Read the model definition and answer for the solid it produces. Units are mm, in the model's axes. A direction names the side the tool comes from. Give positions to 0.01 mm unless a question says otherwise; leave off trailing zeros. Write each loop counter-clockwise with the first axis right and the second up, starting at its lowest first coordinate (ties: lowest second). Pieces come first, ordered by that corner, then holes.
```python
from build123d import *

# Parameters (mm, degrees)
BOSS_EXTRUDE1_DEPTH = 7
SKETCH3_R           = 4.2
SKETCH3_R_2         = 31
CUT_EXTRUDE1_DEPTH  = 156.951680739
SKETCH5_R           = 31
SKETCH5_R_2         = 29.4
BOSS_EXTRUDE3_DEPTH = 2
CUT_EXTRUDE3_DEPTH  = 156.951680739


with BuildPart() as part:
    # Sketch1 → Boss-Extrude1 (new, symmetric)
    with BuildSketch(Plane.XY):
        with BuildLine():
            Line((-41.457265734, 7.66555398), (-63.259986532, -110.249105832))
            ThreePointArc((-63.259986532, -110.249105832), (-57.764447863, -119.708474266), (-47.579981062, -115.713823794))
            Line((-47.579981062, -115.713823794), (-25.616732048, -74.324411645))
            ThreePointArc((-25.616732048, -74.324411645), (-5.909772036, -59.526451333), (18.065040544, -65.231910476))
            Line((18.065040544, -65.231910476), (84.767367566, -118.347513787))
            ThreePointArc((84.767367566, -118.347513787), (95.212080879, -118.36382677), (97.598433891, -108.195364664))
            Line((97.598433891, -108.195364664), (38.136901528, 17.973378699))
            ThreePointArc((38.136901528, 17.973378699), (-5.414703798, 41.810842885), (-41.457265734, 7.66555398))
        make_face()
    extrude(amount=BOSS_EXTRUDE1_DEPTH, both=True)

    # Sketch3 → Cut-Extrude1 (cut, through all)
    with BuildSketch(Plane.XY.offset(7)):
        with Locations((-55, -111.776398371)):
            Circle(SKETCH3_R)
        with Locations((90, -111.776398371)):
            Circle(SKETCH3_R)
        Circle(SKETCH3_R_2)
    extrude(amount=-CUT_EXTRUDE1_DEPTH, mode=Mode.SUBTRACT)

    # Sketch5 → Boss-Extrude3 (add)
    with BuildSketch(Plane.XY.offset(7)):
        Circle(SKETCH5_R)
        Circle(SKETCH5_R_2, mode=Mode.SUBTRACT)
    extrude(amount=-BOSS_EXTRUDE3_DEPTH)

    # Sketch7 → Cut-Extrude3 (cut, through all)
    with BuildSketch(Plane(origin=(0, 0, -7), x_dir=(-1, 0, 0), z_dir=(0, 0, -1))):
        with BuildLine():
            Line((39.416599892, -25.297435332), (51.444133318, -90.345395421))
            ThreePointArc((51.444133318, -90.345395421), (48.99824365, -94.555459787), (44.465461038, -92.777567771))
            Line((44.465461038, -92.777567771), (37.224653842, -79.132375609))
            ThreePointArc((37.224653842, -79.132375609), (25.615584401, -63.184563156), (10.018252925, -51.108700201))
            ThreePointArc((10.018252925, -51.108700201), (6.525820517, -44.233938334), (11.473159104, -38.319272177))
            ThreePointArc((11.473159104, -38.319272177), (23.05966211, -32.684124333), (32.253697166, -23.657958896))
            ThreePointArc((32.253697166, -23.657958896), (36.373945084, -22.123685051), (39.416599892, -25.297435332))
        make_face()
        with BuildLine():
            Line((-47.659866623, -20.998502649), (-79.20248655, -87.927365066))
            ThreePointArc((-79.20248655, -87.927365066), (-77.355903862, -95.795817886), (-69.273685228, -95.783194745))
            Line((-69.273685228, -95.783194745), (-9.558730446, -48.231692548))
            ThreePointArc((-9.558730446, -48.231692548), (-7.514321735, -42.69576591), (-11.473159104, -38.319272177))
            ThreePointArc((-11.473159104, -38.319272177), (-24.638900988, -31.510705453), (-34.421516336, -20.375456146))
            ThreePointArc((-34.421516336, -20.375456146), (-41.228138553, -16.704146639), (-47.659866623, -20.998502649))
        make_face()
    extrude(amount=-CUT_EXTRUDE3_DEPTH, mode=Mode.SUBTRACT)


solid = part.part
```
Item 1: Section B-B (x = 0) is taken. Write down the section's boundary in (y, z), and give its area (3 significant figures).
Result set:
outline: (-58.92, -7) - (-31, -7) - (-31, 5) - (-29.4, 5) - (-29.4, 7) - (-58.92, 7) - close; (29.4, 5) - (31, 5) - (31, -7) - (42.16, -7) - (42.16, 7) - (29.4, 7) - close
area: 553 mm2
Item 2: Which of the six approach directions +Z, -Z, +X, -X, +Y, -Y give full straight-line access (tool end or side, diameter ignored) to faces 1 (the flat face through (50.95, -91.42, 0.1)), 2 (the flat face through (11.3, -27.4, 5)), 3 (the cylindrical face through (7.5, -42.78, -0.1))?
Result set:
face 1: +Z, -Z, -Y
face 2: -Z
face 3: +Z, -Z
Item 3: Determine the mould class of faces 4 (the flat face through (5, -39, -7)), 5 (the flat face through (68.28, -45.99, 0.1)), 6 (the cylindrical face through (41.1, -16.7, -0.1)) for opening direction X: pulls with the +X half, pulls with the -X half, needs draft (parallel to the pull), parting line crosses it, or undercut.
Result set:
face 4: needs draft
face 5: pulls with the +X half
face 6: undercut
Item 4: Section C-C (x = 21) is taken. Write down the section's boundary in (y, z).
Result set:
outline: (-67.57, -7) - (-57.34, -7) - (-57.34, 7) - (-67.57, 7) - close; (-34.04, -7) - (-22.8, -7) - (-22.8, 5) - (-20.58, 5) - (-20.58, 7) - (-34.04, 7) - close; (20.58, 5) - (22.8, 5) - (22.8, -7) - (36.56, -7) - (36.56, 7) - (20.58, 7) - close
Item 5: Find the intervals of material crossed by line 1 along X through (y, z) = (-37, 0.25); line 2 along Y through (x, z) = (11.5, 5.75); line 3 along Y through (x, z) = (0, 0.75), in increasing order.
Result set:
line 1: x = -49.72 to -41.58, -15.2 to 15.2, 55.2 to 64.05
line 2: y = -61.3 to -49.78, -38.31 to -27.06, 27.06 to 40.56
line 3: y = -58.92 to -31, 31 to 42.16
Item 6: Section D-D (y = -36) is taken. Write down the section's boundary in (x, z).
Result set:
outline: (-49.53, -7) - (-41.4, -7) - (-41.4, 7) - (-49.53, 7) - close; (-17.44, -7) - (17.44, -7) - (17.44, 7) - (-17.44, 7) - close; (54.73, -7) - (63.57, -7) - (63.57, 7) - (54.73, 7) - close
Item 7: Section A-A (y = -104) is taken. Write down the section's boundary in (x, z), and give its area (3 significant figures).
Result set:
outline: (-62.1, -7) - (-41.36, -7) - (-41.36, 7) - (-62.1, 7) - close; (66.75, -7) - (95.62, -7) - (95.62, 7) - (66.75, 7) - close
area: 695 mm2
Item 8: Each of these flat-tipped pins is pushed along its axis until it touches: pin 1 Ø6 at (x, z) = (3, -2) entering from -Y; pin 2 Ø1 at (y, z) = (-65, 1.5) entering from +X; pin 3 Ø4 at (y, z) = (-42.5, -1) entering from -X. Where does it stop, or does it pass through?
Result set:
pin 1: stops at y = -59.55
pin 2: stops at x = 77.48
pin 3: stops at x = -51.1
